```python
from build123d import *

# Parameters (mm, degrees)
SKETCH1_W                          = 21.5
SKETCH1_H                          = 21.5
BOSS_EXTRUDE1_DEPTH                = 3.2
SKETCH2_W                          = 5.5
SKETCH2_H                          = 1.2
CUT_EXTRUDE1_DEPTH                 = 27.231822721
SKETCH3_W                          = 21.5
SKETCH3_H                          = 21.5
SKETCH3_W_2                        = 5.5
SKETCH3_H_2                        = 5.5
BOSS_EXTRUDE2_DEPTH                = 0.15
SKETCH11_W                         = 4
SKETCH11_H                         = 4
CUT_EXTRUDE2_DEPTH                 = 19.869717175
TAP_DRILL_FOR_M2X0_4_TAP3_D        = 1.6
TAP_DRILL_FOR_M2_5X0_45_TAP1_D     = 2.05
TAP_DRILL_FOR_M2_5X0_45_TAP1_DEPTH = 1
CUT_EXTRUDE3_REACH                 = 20.896
SKETCH18_W                         = 5.5
SKETCH18_H                         = 5.5
FILLET3_R                          = 1
SKETCH21_W                         = 13.124555245
SKETCH21_H                         = 35.298127434
CUT_EXTRUDE8_DEPTH                 = 19.895733017
SKETCH22_W                         = 0.25
SKETCH22_H                         = 1.2
CUT_EXTRUDE9_DEPTH                 = 27.250543295


with BuildPart() as part:
    # Sketch1 → Boss-Extrude1 (new body)
    with BuildSketch(Plane(origin=(0, 0, 0), x_dir=(1, 0, 0), z_dir=(0, 1, 0))):
        with Locations((-3.933954619, -0.660858995)):
            Rectangle(SKETCH1_W, SKETCH1_H)
    extrude(amount=BOSS_EXTRUDE1_DEPTH)

    # Sketch2 → Cut-Extrude1 (cut, through all)
    with BuildSketch(Plane.XY.offset(11.410858995)):
        with Locations((-3.933954619, 1.6)):
            Rectangle(SKETCH2_W, SKETCH2_H)
    extrude(amount=-CUT_EXTRUDE1_DEPTH, mode=Mode.SUBTRACT)

    # Sketch3 → Boss-Extrude2 (add)
    with BuildSketch(Plane(origin=(0, 3.2, 0), x_dir=(1, 0, 0), z_dir=(0, 1, 0))):
        with Locations((-3.933954619, -0.660858995)):
            Rectangle(SKETCH3_W, SKETCH3_H)
        with Locations((-3.933954619, -0.660858995)):
            Rectangle(SKETCH3_W_2, SKETCH3_H_2, mode=Mode.SUBTRACT)
    extrude(amount=BOSS_EXTRUDE2_DEPTH)

    # Sketch11 → Cut-Extrude2 (cut, through all)
    with BuildSketch(Plane(origin=(0, 3.2, 0), x_dir=(1, 0, 0), z_dir=(0, 1, 0))):
        with Locations((-3.933954619, -0.660858995)):
            Rectangle(SKETCH11_W, SKETCH11_H)
    extrude(amount=-CUT_EXTRUDE2_DEPTH, mode=Mode.SUBTRACT)

    # Tap Drill for M2x0.4 Tap3 (through all)
    with Locations(Plane(origin=(0, 3.35, 0), x_dir=(1, 0, 0), z_dir=(0, 1, 0))):
        with Locations((-12.683954619, 8.089141005), (4.816045381, 8.089141005), (4.816045381, -9.410858995), (-12.683954619, -9.410858995)):
            Hole(TAP_DRILL_FOR_M2X0_4_TAP3_D / 2)

    # Tap Drill for M2.5x0.45 Tap1
    with Locations(Plane(origin=(0, 0, 0), x_dir=(-1, 0, 0), z_dir=(0, -1, 0))):
        with Locations((3.933954619, 8.089141005), (3.933954619, -9.410858995), (3.933954619, 4.539141005), (3.933954619, -5.860858995)):
            Hole(TAP_DRILL_FOR_M2_5X0_45_TAP1_D / 2, depth=TAP_DRILL_FOR_M2_5X0_45_TAP1_DEPTH)

    # Sketch18 → Cut-Extrude3 (cut, up to next)
    with BuildSketch(Plane.XZ, mode=Mode.PRIVATE) as cut_extrude3_sk1:
        with Locations((-3.933954619, 0.660858995)):
            Rectangle(SKETCH18_W, SKETCH18_H)
    cut_extrude3_tool1 = extrude(cut_extrude3_sk1.sketch, amount=-CUT_EXTRUDE3_REACH, mode=Mode.PRIVATE) & part.part
    add(cut_extrude3_tool1.solids().sort_by_distance((-3.933955, 0, 0.660859))[0], mode=Mode.SUBTRACT)

    # Fillet3
    fillet3_edges = [part.edges().sort_by_distance(p)[0] for p in [
        (-14.683954619, 1.675, -10.089141005),
        (6.816045381, 1.675, -10.089141005),
        (6.816045381, 1.675, 11.410858995),
        (-14.683954619, 1.675, 11.410858995),
    ]]
    fillet(fillet3_edges, radius=FILLET3_R)

    # Sketch21 → Cut-Extrude8 (cut, through all)
    with BuildSketch(Plane(origin=(0, 3.35, 0), x_dir=(1, 0, 0), z_dir=(0, 1, 0))):
        with Locations((5.628323004, -1.911462044)):
            Rectangle(SKETCH21_W, SKETCH21_H)
    extrude(amount=-CUT_EXTRUDE8_DEPTH, mode=Mode.SUBTRACT)

    # Sketch22 → Cut-Extrude9 (cut, through all)
    with BuildSketch(Plane(origin=(0, 0, -10.089141005), x_dir=(-1, 0, 0), z_dir=(0, 0, -1))):
        with Locations((1.058954619, 1.6)):
            Rectangle(SKETCH22_W, SKETCH22_H)
    extrude(amount=-CUT_EXTRUDE9_DEPTH, mode=Mode.SUBTRACT)


solid = part.part
```
Geometry: final body of the model. Coordinates: model frame, mm. A direction names the side the tool comes from. Coordinates: 2 decimals unless noted, no trailing zeros. Order: outer loops, then holes, each group sorted by start corner. A loop starts at its lowest first (then second) coordinate and runs counter-clockwise, first axis right, second up. Notation, with made-up numbers: (86, 57.5) - (137, 57.5) arc R16 cw to (137, 68.5) - close; hole circle Ø7 at (52, -35). An arc over 180 degrees is marked (long way). Write each question's results on one line, items separated by ' | '.
1) Set-up query: faces 1 (the flat face through (-6.684, 1, 1)), 2 (the flat face through (-2, 1, -4)), 3 (the flat face through (-4, 3, 2.661)). Return all of +Z, -Z, +X, -X, +Y, -Y with unobstructed straight access to the full face (end or side cutting, diameter ignored); none if empty.
Results list:
face 1: none | face 2: +Z, -Z, +X | face 3: +Y, -Y
2) Section B-B, the plane z = 0.25. Return loops of the section in (x, y).
Results list:
outline: (-14.68, 0) - (-6.68, 0) - (-6.68, 2.2) - (-5.93, 2.2) - (-5.93, 3.2) - (-6.68, 3.2) - (-6.68, 3.35) - (-14.68, 3.35) - close; (-1.93, 2.2) - (-0.93, 2.2) - (-0.93, 3.35) - (-1.18, 3.35) - (-1.18, 3.2) - (-1.93, 3.2) - close; (-1.18, 0) - (-0.93, 0) - (-0.93, 1) - (-1.18, 1) - close
3) Section D-D, the plane z = -5.25. Return loops of the section in (x, y).
Results list:
outline: (-14.68, 0) - (-4.67, 0) - (-4.67, 1) - (-6.68, 1) - (-6.68, 2.2) - (-0.93, 2.2) - (-0.93, 3.35) - (-14.68, 3.35) - close; (-3.2, 0) - (-0.93, 0) - (-0.93, 1) - (-3.2, 1) - close
4) Pin query (flat end, axial travel): pin 1 (1.7 mm diameter, centred on x = -5, z = 3.5, fed in from -Y). Return the tip coordinate at first contact, or that it passes through.
Results list:
pin 1: y = 0
5) Section C-C, the plane x = -13. Return loops of the section in (y, z).
Results list:
outline: (0, -10.09) - (3.35, -10.09) - (3.35, -8.82) - (0, -8.82) - close; (0, -7.35) - (3.35, -7.35) - (3.35, 8.68) - (0, 8.68) - close; (0, 10.15) - (3.35, 10.15) - (3.35, 11.41) - (0, 11.41) - close
6) Line query: line 1 (Z direction, x = -12.75, y = 2.5); line 2 (Y direction, x = -2, z = 9.5); line 3 (Z direction, x = -1.25, y = 0.3). Output: solid intervals per line, ascending. Write a range as from..to.
Results list:
line 1: -10.09..-8.89, -7.29..8.61, 10.21..11.41 | line 2: 0..1, 2.2..3.35 | line 3: -10.09..-2.09, 3.41..11.41
7) Section A-A, the plane x = -2.5. Return loops of the section in (y, z), plus the area to 3 significant figures.
Results list:
outline: (0, -10.09) - (1, -10.09) - (1, -2.09) - (0, -2.09) - close; (0, 3.41) - (1, 3.41) - (1, 11.41) - (0, 11.41) - close; (2.2, -10.09) - (3.35, -10.09) - (3.35, -2.09) - (3.2, -2.09) - (3.2, -1.34) - (2.2, -1.34) - close; (2.2, 2.66) - (3.2, 2.66) - (3.2, 3.41) - (3.35, 3.41) - (3.35, 11.41) - (2.2, 11.41) - close | area: 35.9 mm^2
8) Pull-direction query (Z, two-part tool) for faces 4 (the flat face through (-7, 2, 11.411)), 5 (the flat face through (-4, 0.5, 3.411)), 6 (the flat face through (-14.684, 2, 1)), 7 (the cylindrical face through (-3.38, 0.51, -8.95)); classes: pulls with the +Z half, pulls with the -Z half, needs draft (parallel to the pull), parting line crosses it, or undercut.
Results list:
face 4: pulls with the +Z half | face 5: undercut | face 6: needs draft | face 7: undercut
